Design review of the part shown in the three views and the two pictorial views. Dimensions are in mm from the part's minimum x, y and z. Give positions to 0.01 mm unless a question says otherwise; leave off trailing zeros. Order: outer loops, then holes, each group sorted by start corner. A loop starts at its lowest first (then second) coordinate and runs counter-clockwise, first axis right, second up.
Item 1: Consider section D-D (x = 118). Give the boundary of the cut face in (y, z).
Item 2: Consider section B-B (z = 47). Give the boundary of the cut face in (x, y).
Item 3: Consider section A-A (y = 27). Give the boundary of the cut face in (x, z).
Item 4: Consider section C-C (x = 62.5). Give the boundary of the cut face in (y, z).
Item 5: For probe 1 along X at (y, z) = (26, 19); probe 2 along X at (y, z) = (25.5, 86); probe 3 along Y at (x, z) = (49.5, 76), list the stretches that pass through material, from the lowest coordinate up.
Item 6: For P1, Ø20.5, axis at x = 65.99, y = 27, coming from the +Z side; P2, Ø12.5, axis at x = 91, z = 77, coming from the +Y side; P3, Ø16, axis at x = 276.56, y = 27, coming from the -Z side, all flat-tipped, find the tip position at first contact; note any pin that passes through.
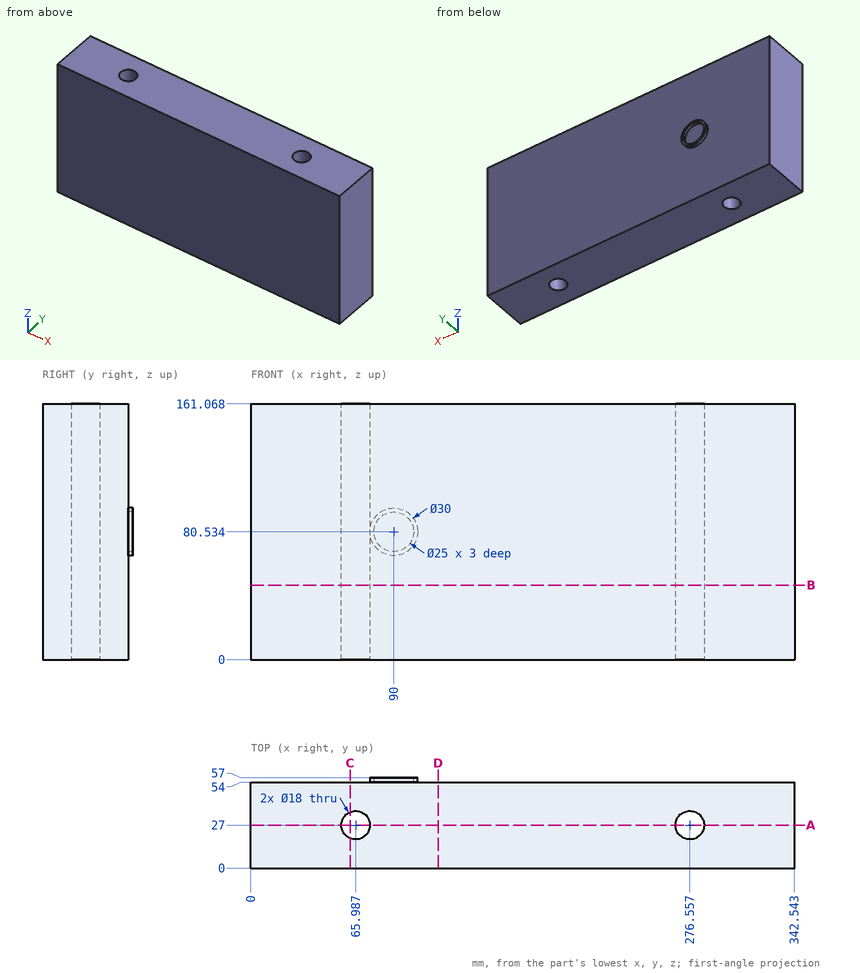
Resolved:
1. outline: (0, 0) - (54, 0) - (54, 161.07) - (0, 161.07) - close
2. outline: (0, 0) - (342.54, 0) - (342.54, 54) - (0, 54) - close; hole circle Ø18 at (65.99, 27); hole circle Ø18 at (276.56, 27)
3. outline: (0, 0) - (56.99, 0) - (56.99, 161.07) - (0, 161.07) - close; (74.99, 0) - (267.56, 0) - (267.56, 161.07) - (74.99, 161.07) - close; (285.56, 0) - (342.54, 0) - (342.54, 161.07) - (285.56, 161.07) - close
4. outline: (0, 0) - (18.7, 0) - (18.7, 161.07) - (0, 161.07) - close; (35.3, 0) - (54, 0) - (54, 161.07) - (35.3, 161.07) - close
5. probe 1: x = 0 to 57.04, 74.93 to 267.61, 285.5 to 342.54
5. probe 2: x = 0 to 57.11, 74.86 to 267.68, 285.43 to 342.54
5. probe 3: y = 0 to 54
6. P1: stops at z = 161.07
6. P2: stops at y = 54
6. P3: passes through
